Model file for the job. Use its own axes, mm. A direction names the side the tool comes from. Round coordinates to 2 decimals unless told otherwise and drop trailing zeros. Write each loop counter-clockwise with the first axis right and the second up, starting at its lowest first coordinate (ties: lowest second). Pieces come first, ordered by that corner, then holes. Notation, with made-up numbers: (34.5, -29.5) - (39.5, -29.5) arc R22 ccw to (39.5, -21.5) - close; hole circle Ø2 at (-21.75, 27.25). An arc over 180 degrees is marked (long way). Answer as a JSON object with one key per item and string values. Group by question number.
from build123d import *

# Parameters (mm, degrees)
BOSS_EXTRU_1_DEPTH      = 1.5
ESQUISSE2_R             = 1.75
ENL_V_MAT_EXTRU_1_DEPTH = 20.139292045
ESQUISSE3_R             = 0.65
BOSS_EXTRU_2_DEPTH      = 2
ESQUISSE4_R             = 0.15
BOSS_EXTRU_3_DEPTH      = 4
ESQUISSE6_R             = 1
ENL_V_MAT_EXTRU_2_DEPTH = 20.857303442


with BuildPart() as part:
    # Esquisse1 → Boss.-Extru.1 (new body)
    with BuildSketch(Plane(origin=(0, 0, 0), x_dir=(1, 0, 0), z_dir=(0, 1, 0))):
        with BuildLine():
            Line((-5, 8.660254038), (-14.375, 3.247595264))
            ThreePointArc((-14.375, 3.247595264), (-16.25, 0), (-14.375, -3.247595264))
            Line((-14.375, -3.247595264), (-5, -8.660254038))
            ThreePointArc((-5, -8.660254038), (0, -10), (5, -8.660254038))
            Line((5, -8.660254038), (14.375, -3.247595264))
            ThreePointArc((14.375, -3.247595264), (16.25, 0), (14.375, 3.247595264))
            Line((14.375, 3.247595264), (5, 8.660254038))
            ThreePointArc((5, 8.660254038), (0, 10), (-5, 8.660254038))
        make_face()
    extrude(amount=BOSS_EXTRU_1_DEPTH)

    # Esquisse2 → Enlèv. mat.-Extru.1 (cut, through all)
    with BuildSketch(Plane(origin=(0, 1.5, 0), x_dir=(1, 0, 0), z_dir=(0, 1, 0))):
        with Locations(Location((-12.5, 0, 0), (0, 0, 270))):
            Circle(ESQUISSE2_R)
        with Locations(Location((12.5, 0, 0), (0, 0, 270))):
            Circle(ESQUISSE2_R)
    extrude(amount=-ENL_V_MAT_EXTRU_1_DEPTH, mode=Mode.SUBTRACT)

    # Esquisse3 → Boss.-Extru.2 (add)
    with BuildSketch(Plane(origin=(0, 1.5, 0), x_dir=(1, 0, 0), z_dir=(0, 1, 0))):
        with Locations(Location((6.15, 0, 0), (0, 0, 270))):
            Circle(ESQUISSE3_R)
        with Locations(Location((5.445554558, -2.858047508, 0), (0, 0, 270))):
            Circle(ESQUISSE3_R)
        with Locations(Location((3.493598192, -5.061350775, 0), (0, 0, 270))):
            Circle(ESQUISSE3_R)
        with Locations(Location((0.741300584, -6.105159576, 0), (0, 0, 270))):
            Circle(ESQUISSE3_R)
        with Locations(Location((-2.180820055, -5.750349893, 0), (0, 0, 270))):
            Circle(ESQUISSE3_R)
        with Locations(Location((-4.603341101, -4.078204348, 0), (0, 0, 270))):
            Circle(ESQUISSE3_R)
        with Locations(Location((-5.971292177, -1.471791335, 0), (0, 0, 270))):
            Circle(ESQUISSE3_R)
        with Locations(Location((-5.971292177, 1.471791335, 0), (0, 0, 270))):
            Circle(ESQUISSE3_R)
        with Locations(Location((-4.603341101, 4.078204348, 0), (0, 0, 270))):
            Circle(ESQUISSE3_R)
        with Locations(Location((-2.180820055, 5.750349893, 0), (0, 0, 270))):
            Circle(ESQUISSE3_R)
        with Locations(Location((0.741300584, 6.105159576, 0), (0, 0, 270))):
            Circle(ESQUISSE3_R)
        with Locations(Location((3.493598192, 5.061350775, 0), (0, 0, 270))):
            Circle(ESQUISSE3_R)
        with Locations(Location((5.445554558, 2.858047508, 0), (0, 0, 270))):
            Circle(ESQUISSE3_R)
    extrude(amount=BOSS_EXTRU_2_DEPTH)

    # Esquisse4 → Boss.-Extru.3 (add)
    with BuildSketch(Plane.XZ):
        with Locations(Location((6.15, 0, 0), (0, 0, 90))):
            Circle(ESQUISSE4_R)
        with Locations(Location((5.445554558, -2.858047508, 0), (0, 0, 90))):
            Circle(ESQUISSE4_R)
        with Locations(Location((3.493598192, -5.061350775, 0), (0, 0, 90))):
            Circle(ESQUISSE4_R)
        with Locations(Location((0.741300584, -6.105159576, 0), (0, 0, 90))):
            Circle(ESQUISSE4_R)
        with Locations(Location((-2.180820055, -5.750349893, 0), (0, 0, 90))):
            Circle(ESQUISSE4_R)
        with Locations(Location((-4.603341101, -4.078204348, 0), (0, 0, 90))):
            Circle(ESQUISSE4_R)
        with Locations(Location((-5.971292177, -1.471791335, 0), (0, 0, 90))):
            Circle(ESQUISSE4_R)
        with Locations(Location((-5.971292177, 1.471791335, 0), (0, 0, 90))):
            Circle(ESQUISSE4_R)
        with Locations(Location((-4.603341101, 4.078204348, 0), (0, 0, 90))):
            Circle(ESQUISSE4_R)
        with Locations(Location((-2.180820055, 5.750349893, 0), (0, 0, 90))):
            Circle(ESQUISSE4_R)
        with Locations(Location((0.741300584, 6.105159576, 0), (0, 0, 90))):
            Circle(ESQUISSE4_R)
        with Locations(Location((3.493598192, 5.061350775, 0), (0, 0, 90))):
            Circle(ESQUISSE4_R)
        with Locations(Location((5.445554558, 2.858047508, 0), (0, 0, 90))):
            Circle(ESQUISSE4_R)
    extrude(amount=BOSS_EXTRU_3_DEPTH)

    # Esquisse6 → Enlèv. mat.-Extru.2 (cut, through all)
    with BuildSketch(Plane(origin=(0, 1.5, 0), x_dir=(1, 0, 0), z_dir=(0, 1, 0))):
        with Locations(Location((0, 0, 0), (0, 0, 270))):
            Circle(ESQUISSE6_R)
    extrude(amount=-ENL_V_MAT_EXTRU_2_DEPTH, mode=Mode.SUBTRACT)


solid = part.part
(1) Pull direction X, two halves, no side cores. Call faces 1 (the cylindrical face through (-16.25, 0.74, -0.05)), 2 (the cylindrical face through (-10.765, 0.76, -0.228)), 3 (the flat face through (9.622, 0.74, 5.992)), 4 (the flat face through (-2, 3.5, -6)): pulls with the +X half, pulls with the -X half, needs draft (parallel to the pull), parting line crosses it, or undercut.
(2) Slice it at A-A (y = -0.5). Count the separate pieces of the cut face and the enclosed holes in it, then the cut area to 3 significant figures.
(3) Slice it at C-C (y = 1). Write the cut outline in (x, z) (3 decimals), then the cut area to 3 significant figures.
(4) Drill centre lines: line 1 (Y direction, x = 5, z = -7.5); line 2 (X direction, y = 2.5, z = 4); line 3 (Z direction, x = 1, y = 2.25). Where is each one in solid material? Low to high. Write a range as from..to.
(5) Slice it at D-D (x = -12). Write the cut outline in (y, z), then the cut area to 3 significant figures.
(6) Slice it at B-B (x = 12.5). Write the cut outline in (y, z), then the cut area to 3 significant figures.
(7) Flat gauge pins, fed straight in: pin 1 (2 mm diameter, centred on x = -5, z = 1.5, fed in from -Y); pin 2 (2 mm diameter, centred on x = -12.5, z = 0, fed in from +Y); pin 3 (1 mm diameter, centred on x = 2, z = 1.5, fed in from -Y); pin 4 (8 mm diameter, centred on x = 10.5, z = -3.5, fed in from +Y). Where does each tip first touch, or does it go through?
(8) 3-axis set-ups, long thin cutter, end or side, ignore diameter. For faces 5 (the cylindrical face through (16.25, 0.74, 0.05)), 6 (the cylindrical face through (0.77, 2.486, -6.755)): which of +Z, -Z, +X, -X, +Y, -Y reach the whole face in a straight line?
Answer:
{
 "1": {"face 1": "pulls with the -X half", "face 2": "undercut", "face 3": "pulls with the +X half", "face 4": "needs draft"},
 "2": {"separate pieces": "13", "enclosed holes": "0", "area": "0.919 mm²"},
 "3": {"outline": "(-14.375, -3.248) - (-5, -8.66) arc R10 ccw to (5, -8.66) - (14.375, -3.248) arc R3.75 ccw to (14.375, 3.248) - (5, 8.66) arc R10 ccw to (-5, 8.66) - (-14.375, 3.248) arc R3.75 ccw to start; hole circle Ø3.5 at (-12.5, 0); hole circle Ø2 at (0, 0); hole circle Ø3.5 at (12.5, 0)", "area": "409 mm²"},
 "4": {"line 1": "0..1.5", "line 2": "-5.25..-3.96", "line 3": "-6.7..-5.51, 5.51..6.7"},
 "5": {"outline": "(0, -4.62) - (1.5, -4.62) - (1.5, -1.68) - (0, -1.68) - close; (0, 1.68) - (1.5, 1.68) - (1.5, 4.62) - (0, 4.62) - close", "area": "8.83 mm²"},
 "6": {"outline": "(0, -4.33) - (1.5, -4.33) - (1.5, -1.75) - (0, -1.75) - close; (0, 1.75) - (1.5, 1.75) - (1.5, 4.33) - (0, 4.33) - close", "area": "7.74 mm²"},
 "7": {"pin 1": "y = -4", "pin 2": "through", "pin 3": "y = 0", "pin 4": "y = 1.5"},
 "8": {"face 5": "+X, +Y, -Y", "face 6": "+Y"}
}
